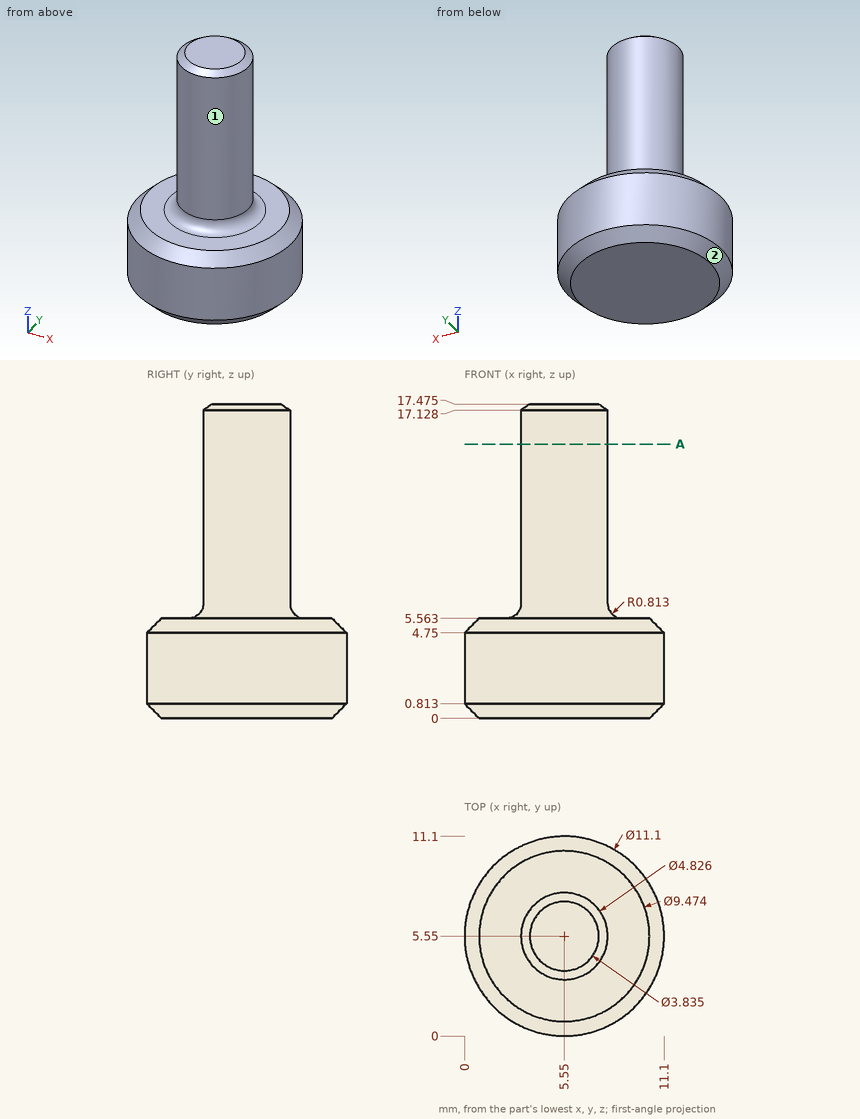
Can you work these out from the drawing? Everything is in mm from the part's minimum corner. A direction names the side the tool comes from. Give positions to 0.01 mm unless a question says otherwise; leave off trailing zeros. Order: outer loops, then holes, each group sorted by start corner. A loop starts at its lowest first (then second) coordinate and runs counter-clockwise, first axis right, second up. Notation, with made-up numbers: M 57.5,-10 L 67.5,-10 A21 cw 67.5,27 Z; hole C 0,47.25 d10. An arc over 180 degrees is marked long. Use a Markdown table: item, result. Add a question column.
1. On a 3-axis mill with a long thin cutter (end or side, diameter ignored), from which of +Z, -Z, +X, -X, +Y, -Y can I reach the whole of each face in a straight line? I mean the marked faces 1 and 2. Say none if no direction works.
2. Suppose I cut it at A-A (z = 15.25). List the corners of the cut face in (x, y) for me.
3. I need wall thicknesses on probe 1 along Z at (x, y) = (1.5, 5.5); probe 2 along Z at (x, y) = (10.25, 4); probe 3 along X at (y, z) = (7.5, 3.75) (1 decimal). Which ranges of each line are inside material? Lowest first, please. Write a range as from..to.
4. For pin 1 Ø2 at (y, z) = (2.5, 2) entering from -X; pin 2 Ø1 at (x, z) = (7, 5) entering from -Y; pin 3 Ø5 at (x, z) = (3, 11) entering from -Y; pin 4 Ø1 at (y, z) = (8.5, 15.5) entering from +X, each with a flat end and sliding along its axis, tell me the tip position at first contact or that it passes through.
Results list:
| question | item | result |
|---|---|---|
| 1 | face 1 | +Z |
| 1 | face 2 | -Z |
| 2 | outline | C 5.55,5.55 d4.83 |
| 3 | probe 1 | z = 0..5.56 |
| 3 | probe 2 | z = 0.21..5.35 |
| 3 | probe 3 | x = 0.4..10.7 |
| 4 | pin 1 | stops at x = 0.39 |
| 4 | pin 2 | stops at y = 0.09 |
| 4 | pin 3 | stops at y = 3.14 |
| 4 | pin 4 | passes through |
